Build history of the part. All positions in model axes, mm. Coordinates: 2 decimals unless noted, no trailing zeros. One line per item, written item: value.
```python
from build123d import *

# Parameters (mm, degrees)
SKETCH011_W      = 121.654072
SKETCH011_H      = 73.26893
PAD009_DEPTH     = 4
HOLE_D           = 3
HOLE_DEPTH       = 25
HOLE_CSINK_D     = 6.9
HOLE_CSINK_ANGLE = 90
CHAMFER_SIZE     = 5


with BuildPart() as part:
    # Sketch011 → Pad009 (new body)
    with BuildSketch(Plane.YZ):
        with Locations((0.298689, 17.336089)):
            Rectangle(SKETCH011_W, SKETCH011_H)
    extrude(amount=PAD009_DEPTH)

    # Hole
    with Locations(Plane.YZ.offset(4)):
        with Locations((-31.394375, 43.94352), (32.693371, -12.187573)):
            CounterSinkHole(HOLE_D / 2, HOLE_CSINK_D / 2, depth=HOLE_DEPTH, counter_sink_angle=HOLE_CSINK_ANGLE)

    # Chamfer
    chamfer_edges = [part.edges().sort_by_distance(p)[0] for p in [
        (2, -60.528347, 53.970554),
        (2, 61.125725, 53.970554),
        (2, -60.528347, -19.298376),
        (2, 61.125725, -19.298376),
    ]]
    chamfer(chamfer_edges, length=CHAMFER_SIZE)


with BuildPart() as part_1:
    # Body004 placement: moved
    add(part.part.moved(Location((32, 0, 0))))


solid = part_1.part
```
Item 1: Probe probe 1 along Y at (x, z) = (35.75, -10.5); probe 2 along Y at (x, z) = (35.1, 51); probe 3 along Z at (x, y) = (32.65, 56.5). List the from-to ranges inside material, lowest first. Write a range as from..to.
Check result:
probe 1: y = -60.53..29.97, 35.41..61.13
probe 2: y = -58.5..59.1
probe 3: z = -18.92..53.6
Item 2: Drop a flat-ended pin along its axis: P1, Ø3.5, axis at y = 32.69, z = -12.19, coming from the +X side. Give the stop position or say it passes through.
Check result:
P1: stops at x = 34.3
Item 3: Pull direction Z, two halves, no side cores. Call faces 1 (the face through (32, -1, 18)), 2 (the face through (33.01, 31.26, -11.74)), 3 (the face through (33.01, -32.2, 45.21)), 4 (the face through (33.972, -57.993, -16.833)): released by +Z, released by -Z, zero draft, split by the parting line, or undercut.
Check result:
face 1: zero draft
face 2: undercut
face 3: undercut
face 4: released by -Z
